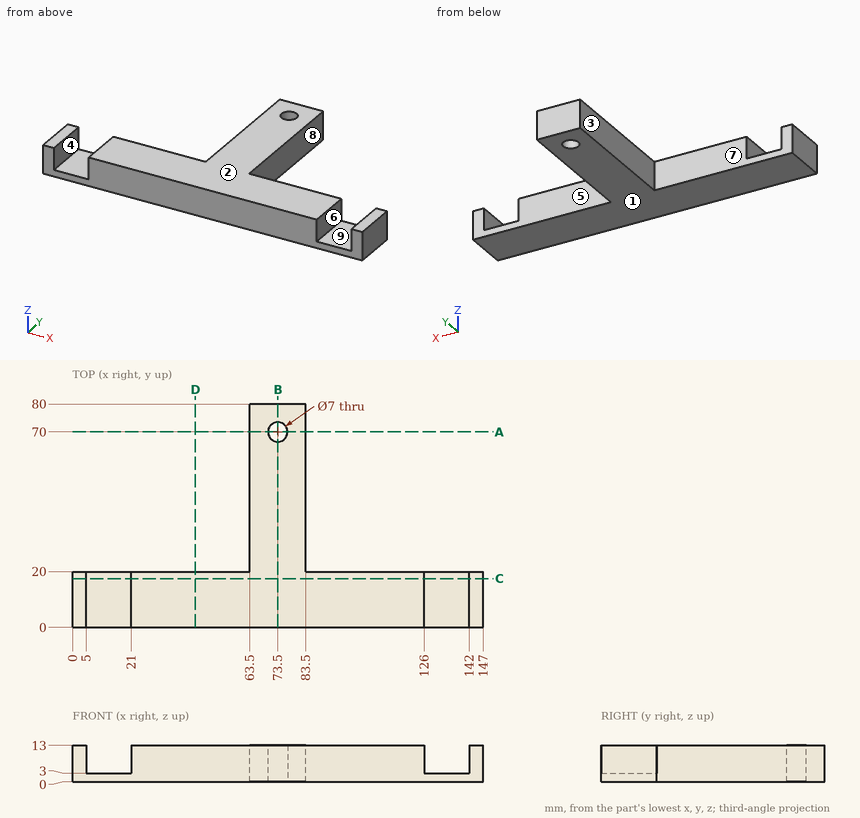
The drawing under review shows one solid part. Ordinate dimensions are in mm from its lowest x, y, z. A direction names the side the tool comes from. Round coordinates to 2 decimals unless told otherwise and drop trailing zeros. Order: outer loops, then holes, each group sorted by start corner. A loop starts at its lowest first (then second) coordinate and runs counter-clockwise, first axis right, second up. Notation, with made-up numbers: (62, 66) -> (114, 66) arc R24 cw to (114, 100) -> close; hole circle Ø10 at (-39, 5). An arc over 180 degrees is marked (long way). Return JSON: item names as keys, results as strings.
1. Insertion check: P1, Ø1.5, axis at y = 53, z = 10, coming from the +X side; P2, Ø8, axis at x = 73.5, y = 70, coming from the +Z side; P3, Ø6, axis at x = 91.5, z = 7, coming from the +Y side; P4, Ø6.5, axis at y = 62.5, z = 9, coming from the -X side. Each pin has a flat end and moves straight along its axis. Give the tip position at first contact, or say it passes through.
Answer block:
{"P1": "stops at x = 83.5", "P2": "stops at z = 13", "P3": "stops at y = 20", "P4": "stops at x = 63.5"}
2. Take a section at A-A (y = 70). Write out the cut boundary in (x, z).
Answer block:
{"outline": "(63.5, 0) -> (70, 0) -> (70, 13) -> (63.5, 13) -> close; (77, 0) -> (83.5, 0) -> (83.5, 13) -> (77, 13) -> close"}
3. For the marked faces 1, 2, 3, 4 and 5, list the 3-axis set-ups (+Z, -Z, +X, -X, +Y, -Y) from which the entire face can be reached by the end or side of a thin tool; tool diameter is ignored.
Answer block:
{"face 1": "-Z, +X, -X, +Y, -Y", "face 2": "+Z, +X, -X, +Y, -Y", "face 3": "+Z, -Z, -X, +Y", "face 4": "+Z, +Y, -Y", "face 5": "+Z, -Z, +X, +Y"}
4. For L1, parallel to X at y = 3.5, z = 8; L2, parallel to Y at x = 73.5, z = 7.5; L3, parallel to Y at x = 26.5, z = 8.25, list the stretches that pass through material, from the lowest coordinate up. Write a range as [from, to].
Answer block:
{"L1": "x = [0, 5], [21, 126], [142, 147]", "L2": "y = [0, 66.5], [73.5, 80]", "L3": "y = [0, 20]"}
5. Take a section at C-C (y = 17.5). Write out the cut boundary in (x, z), then the cut area to 3 significant figures.
Answer block:
{"outline": "(0, 0) -> (147, 0) -> (147, 13) -> (142, 13) -> (142, 3) -> (126, 3) -> (126, 13) -> (21, 13) -> (21, 3) -> (5, 3) -> (5, 13) -> (0, 13) -> close", "area": "1,590 mm²"}
6. The part is to be moulded in two halves that separate along X. For the marked faces 6, 7, 8 and 9, say which applies: +X half, -X half, draft (parallel to the pull), parting line (faces both ways), or undercut.
Answer block:
{"face 6": "undercut", "face 7": "draft", "face 8": "+X half", "face 9": "undercut"}
7. Take a section at B-B (x = 73.5). Write out the cut boundary in (y, z), then the cut area to 3 significant figures.
Answer block:
{"outline": "(0, 0) -> (66.5, 0) -> (66.5, 13) -> (0, 13) -> close; (73.5, 0) -> (80, 0) -> (80, 13) -> (73.5, 13) -> close", "area": "949 mm²"}
8. Take a section at D-D (x = 44). Write out the cut boundary in (y, z).
Answer block:
{"outline": "(0, 0) -> (20, 0) -> (20, 13) -> (0, 13) -> close"}
